from build123d import *

# Parameters (mm, degrees)
F1_DEPTH = 2425
F2_R     = 12
F2_R_2   = 7
F2_R_3   = 9
F3_DEPTH = 10
F4_R     = 7
F5_DEPTH = 10
F6_R     = 20


with BuildPart() as f1:
    # F0 (on Right) → F1 (new body)
    with BuildSketch(Plane.YZ):
        Polygon((-125, 0), (0, 0), (0, 75), (-10, 75), (-10, 10), (-125, 10), align=None)
    extrude(amount=F1_DEPTH)

    # F2 (on face) → F3 (cut)
    with BuildSketch(Plane.XY.offset(10)):
        with Locations((40, -70)):
            Circle(F2_R)
        with Locations((2385, -70)):
            Circle(F2_R)
        with BuildLine():
            Line((1147.5, -125), (1277.5, -125))
            ThreePointArc((1277.5, -125), (1212.5, -100), (1147.5, -125))
        make_face()
        with Locations((1147.5, -100)):
            Circle(F2_R_2)
        with Locations((1277.5, -100)):
            Circle(F2_R_2)
        with Locations((2085, -70)):
            Circle(F2_R_3)
        with Locations((340, -70)):
            Circle(F2_R_3)
    extrude(amount=-F3_DEPTH, mode=Mode.SUBTRACT)

    # F4 (on face) → F5 (cut)
    with BuildSketch(Plane.XZ.offset(10)):
        with Locations((1195, 37.5)):
            Circle(F4_R)
        with Locations((1230, 37.5)):
            Circle(F4_R)
    extrude(amount=-F5_DEPTH, mode=Mode.SUBTRACT)

    # F6
    f6_edges = [f1.edges().sort_by_distance(p)[0] for p in [
        (2425, -5, 75),
        (0, -5, 75),
    ]]
    fillet(f6_edges, radius=F6_R)


solid = f1.part
Verification items for the finished model (mm, model axes). A direction names the side the tool comes from. Round coordinates to 2 decimals unless told otherwise and drop trailing zeros. Loops run counter-clockwise (first coordinate to the right, second up) from the corner with the lowest first, then second, coordinate; pieces in that order, holes last. Notation, with made-up numbers: M -11,19.25 L 15,19.25 A15 cw 15,48.25 Z; hole C -2.5,-28 d7. An arc over 180 degrees is marked long. Write each question's results on one line, items separated by ' | '.
1) Access from +Z, -Z, +X, -X, +Y, -Y to the whole of each face (thin tool, end or side, straight path). Record for faces 1 (the flat face through (0, -49, 9)), 2 (the flat face through (1196, -67, 10)).
Checks:
face 1: +Z, -Z, -X, +Y, -Y | face 2: +Z, +X, -X, -Y
2) Section check B-B on x = 1426. Record the boundary of the cut face in (y, z).
Checks:
outline: M -125,0 L 0,0 L 0,75 L -10,75 L -10,10 L -125,10 Z
3) Scan lines: L1, parallel to Y at x = 40, z = 7; L2, parallel to Z at x = 1195, y = -3; L3, parallel to Z at x = 2178, y = -22. Record each from-to range of solid material in increasing order. Write a range as from..to.
Checks:
L1: y = -125..-82, -58..0 | L2: z = 0..30.5, 44.5..75 | L3: z = 0..10
4) Gauge pin test, flat ends, axial feed: P1, Ø18, axis at x = 1230, z = 37.5, coming from the -Y side; P2, Ø23.5, axis at x = 340, y = -70, coming from the +Z side. Record the tip position at first contact, or that the pin passes through.
Checks:
P1: stops at y = -10 | P2: stops at z = 10
5) Section check A-A on y = -31. Record the boundary of the cut face in (x, z).
Checks:
outline: M 0,0 L 2425,0 L 2425,10 L 0,10 Z
